from build123d import *

# Parameters (mm, degrees)
ESBO_O1_R                = 2
RESSALTO_EXTRUS_O1_DEPTH = 3
ESBO_O2_W                = 44.3
ESBO_O2_H                = 3
RESSALTO_EXTRUS_O2_DEPTH = 10
ESBO_O3_R                = 1.25
ESBO_O3_W                = 16
ESBO_O3_H                = 8
CORTE_EXTRUS_O1_DEPTH    = 3


with BuildPart() as part:
    # Esboço1 → Ressalto-extrusão1 (new body)
    with BuildSketch(Plane(origin=(0, 0, 0), x_dir=(1, 0, 0), z_dir=(0, 1, 0))):
        Polygon((22.15, 5.76), (7.5, 5.76), (7.5, 0), (-7.5, 0), (-7.5, 5.76), (-22.15, 5.76), (-22.15, -5.76), (22.15, -5.76), align=None)
        with Locations(Location((-16.9, 1.76, 0), (0, 0, 270))):
            Circle(ESBO_O1_R, mode=Mode.SUBTRACT)
        with Locations(Location((16.9, 1.76, 0), (0, 0, 90))):
            Circle(ESBO_O1_R, mode=Mode.SUBTRACT)
    extrude(amount=RESSALTO_EXTRUS_O1_DEPTH)

    # Esboço2 → Ressalto-extrusão2 (add)
    with BuildSketch(Plane(origin=(0, 0, 0), x_dir=(-1, 0, 0), z_dir=(0, -1, 0))):
        with Locations((0, -4.26)):
            Rectangle(ESBO_O2_W, ESBO_O2_H)
    extrude(amount=RESSALTO_EXTRUS_O2_DEPTH)

    # Esboço3 → Corte-extrusão1 (cut)
    with BuildSketch(Plane.XY.offset(5.76)):
        with Locations((-9.7, -7.5)):
            Circle(ESBO_O3_R)
        with Locations((9.7, -7.5)):
            Circle(ESBO_O3_R)
        with Locations((0, -6)):
            Rectangle(ESBO_O3_W, ESBO_O3_H)
    extrude(amount=-CORTE_EXTRUS_O1_DEPTH, mode=Mode.SUBTRACT)


solid = part.part
Part model, mm, in its own coordinate system. A direction names the side the tool comes from. Coordinates: 2 decimals unless noted, no trailing zeros. Order: outer loops, then holes, each group sorted by start corner. A loop starts at its lowest first (then second) coordinate and runs counter-clockwise, first axis right, second up. Notation, with made-up numbers: M 49,-31.5 L 104,-31.5 A31 ccw 104,0.5 Z; hole C 61.25,74.25 d7. An arc over 180 degrees is marked long. One line per question, with ' | ' between items.
Q1. Two-plate mould, pull along Z, no slides. Class faces 1 (the face through (-22.15, -1, 4)), 2 (the face through (0, -1, 5.76)), 3 (the face through (-16.299, 1.479, 0.148)): +Z half, -Z half, draft (parallel to the pull), parting line (faces both ways), or undercut.
A:
face 1: draft | face 2: +Z half | face 3: undercut
Q2. Drill centre lines: line 1 (Y direction, x = 9.7, z = 4.7); line 2 (Z direction, x = 16.9, y = 2.2); line 3 (Z direction, x = 18, y = -3.25). Where is each one in solid material? Low to high.
A:
line 1: y = -10 to -8.75, -6.25 to 3 | line 2: z = -5.76 to -3.76, 0.24 to 5.76 | line 3: z = 2.76 to 5.76
Q3. Pin check, flat tips, straight feed: P1, Ø6, axis at x = 7, z = -0.5, coming from the -Y side; P2, Ø1.5, axis at x = 2, z = 4, coming from the -Y side; P3, Ø1.5, axis at x = -0.5, y = 1, coming from the -Z side. Stop position of each tip, or through.
A:
P1: stops at y = 0 | P2: stops at y = -2 | P3: stops at z = 0
Q4. Slice it at C-C (x = 9.7). Give the cut face in (y, z).
A:
outline: M -10,2.76 L -8.75,2.76 L -8.75,5.76 L -10,5.76 Z; M -6.25,2.76 L 0,2.76 L 0,-5.76 L 3,-5.76 L 3,5.76 L -6.25,5.76 Z
Q5. Slice it at A-A (z = -4.5). Give the cut face in (x, y).
A:
outline: M -22.15,0 L -7.5,0 L -7.5,3 L -22.15,3 Z; M 7.5,0 L 22.15,0 L 22.15,3 L 7.5,3 Z
Q6. 3-axis set-ups, long thin cutter, end or side, ignore diameter. For faces 4 (the face through (0, -2, 4)), 5 (the face through (-0.3, 0, 0.3)), 6 (the face through (-7.5, 1, -3)): which of +Z, -Z, +X, -X, +Y, -Y reach the whole face in a straight line?
A:
face 4: +Z, -Z, -Y | face 5: -Z, +X, -X, -Y | face 6: -Z, +Y, -Y
Q7. Slice it at B-B (y = -7.5). Give the cut face in (x, z), and give its area (3 significant figures).
A:
outline: M -22.15,2.76 L -10.95,2.76 L -10.95,5.76 L -22.15,5.76 Z; M -8.45,2.76 L -8,2.76 L -8,5.76 L -8.45,5.76 Z; M 8,2.76 L 8.45,2.76 L 8.45,5.76 L 8,5.76 Z; M 10.95,2.76 L 22.15,2.76 L 22.15,5.76 L 10.95,5.76 Z | area: 69.9 mm^2
Q8. Slice it at D-D (y = -3). Give the cut face in (x, z), and give its area (3 significant figures).
A:
outline: M -22.15,2.76 L -8,2.76 L -8,5.76 L -22.15,5.76 Z; M 8,2.76 L 22.15,2.76 L 22.15,5.76 L 8,5.76 Z | area: 84.9 mm^2
